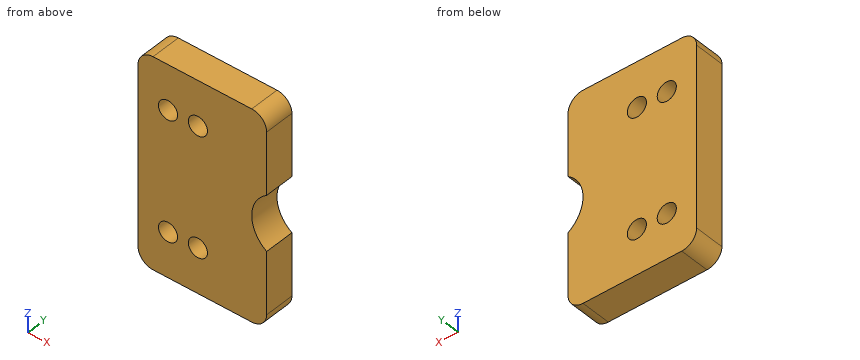
from build123d import *

# Parameters (mm, degrees)
SKETCH1_R           = 4.064
BOSS_EXTRUDE1_DEPTH = 12.7
FILLET1_R           = 6.35


with BuildPart() as part:
    # Sketch1 → Boss-Extrude1 (new body)
    with BuildSketch(Plane(origin=(0, 0, 0), x_dir=(1, 0, 0), z_dir=(0, 1, 0))):
        with BuildLine():
            Line((54.61, 32.741178539), (54.61, 0))
            Line((54.61, 0), (0, 0))
            Line((0, 0), (0, 88.9))
            Line((0, 88.9), (54.61, 88.9))
            Line((54.61, 88.9), (54.61, 56.158821461))
            ThreePointArc((54.61, 56.158821461), (48.26, 44.45), (54.61, 32.741178539))
        make_face()
        with Locations(Location((12.7, 69.85, 0), (0, 0, 270))):
            Circle(SKETCH1_R, mode=Mode.SUBTRACT)
        with Locations(Location((25.4, 69.85, 0), (0, 0, 270))):
            Circle(SKETCH1_R, mode=Mode.SUBTRACT)
        with Locations(Location((25.4, 19.05, 0), (0, 0, 90))):
            Circle(SKETCH1_R, mode=Mode.SUBTRACT)
        with Locations(Location((12.7, 19.05, 0), (0, 0, 90))):
            Circle(SKETCH1_R, mode=Mode.SUBTRACT)
    extrude(amount=BOSS_EXTRUDE1_DEPTH)

    # Fillet1
    fillet1_edges = [part.edges().sort_by_distance(p)[0] for p in [
        (0, 6.35, -88.9),
        (54.61, 6.35, -88.9),
        (54.61, 6.35, 0),
        (0, 6.35, 0),
    ]]
    fillet(fillet1_edges, radius=FILLET1_R)


solid = part.part
Verification items for the finished model (mm, model axes). Coordinates: 2 decimals unless noted, no trailing zeros. Order: outer loops, then holes, each group sorted by start corner. A loop starts at its lowest first (then second) coordinate and runs counter-clockwise, first axis right, second up. Notation, with made-up numbers: (-32, 32.5) -> (-21, 32.5) arc R30 cw to (-21, 65.5) -> close; hole circle Ø5 at (66, -21.75). An arc over 180 degrees is marked (long way). Put each result on its own line as item: value. Start each with the question number.
1. Go/stop test with a flat-tipped pin: pin 1 Ø7.5 at (x, z) = (25.4, -19.05) entering from -Y. Record where the tip stops, or that it passes through.
2. Cross-section at C-C, the plane y = 2.5. Record the boundary of the cut face in (x, z), then the cut area to 3 significant figures.
3. Cross-section at A-A, the plane x = 12.7. Record the boundary of the cut face in (y, z), then the cut area to 3 significant figures.
4. Cross-section at B-B, the plane z = -69.85. Record the boundary of the cut face in (x, y), then the cut area to 3 significant figures.
5. Material ranges on L1, parallel to X at y = 5.75, z = -19.05; L2, parallel to X at y = 9.5, z = -20; L3, parallel to Z at x = 22.5, y = 2.5, recorded low to high. Write a range as [from, to].
6. Cross-section at D-D, the plane z = -54. Record the boundary of the cut face in (x, y).
Computed:
1. pin 1: through
2. outline: (0, -82.55) arc R6.35 ccw to (6.35, -88.9) -> (48.26, -88.9) arc R6.35 ccw to (54.61, -82.55) -> (54.61, -56.16) arc R13.97 cw to (54.61, -32.74) -> (54.61, -6.35) arc R6.35 ccw to (48.26, 0) -> (6.35, 0) arc R6.35 ccw to (0, -6.35) -> close; hole circle Ø8.13 at (12.7, -69.85); hole circle Ø8.13 at (12.7, -19.05); hole circle Ø8.13 at (25.4, -69.85); hole circle Ø8.13 at (25.4, -19.05)
2. area: 4,510 mm2
3. outline: (0, -88.9) -> (12.7, -88.9) -> (12.7, -73.91) -> (0, -73.91) -> close; (0, -65.79) -> (12.7, -65.79) -> (12.7, -23.11) -> (0, -23.11) -> close; (0, -14.99) -> (12.7, -14.99) -> (12.7, 0) -> (0, 0) -> close
3. area: 923 mm2
4. outline: (0, 0) -> (8.64, 0) -> (8.64, 12.7) -> (0, 12.7) -> close; (16.76, 0) -> (21.34, 0) -> (21.34, 12.7) -> (16.76, 12.7) -> close; (29.46, 0) -> (54.61, 0) -> (54.61, 12.7) -> (29.46, 12.7) -> close
4. area: 487 mm2
5. L1: [0, 8.64], [16.76, 21.34], [29.46, 54.61]
5. L2: [0, 8.75], [16.65, 21.45], [29.35, 54.61]
5. L3: [-88.9, -72.7], [-67, -21.9], [-16.2, 0]
6. outline: (0, 0) -> (52.03, 0) -> (52.03, 12.7) -> (0, 12.7) -> close
